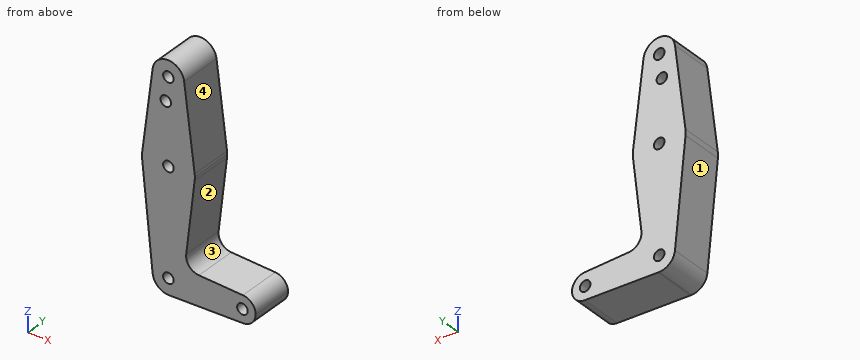
from build123d import *

# Parameters (mm, degrees)
F0_R     = 3.175
F1_DEPTH = 25.4


with BuildPart() as f1:
    # F0 (on Front) → F1 (new body)
    with BuildSketch(Plane.XZ):
        with BuildLine():
            ThreePointArc((15.769913, -1.823585), (15.848707, -0.913305), (15.875, 0))
            ThreePointArc((15.875, 0), (15.843841, 0.994139), (15.750488, 1.984375))
            ThreePointArc((15.750488, 1.984375), (0, 15.875), (-15.750488, 1.984375))
            ThreePointArc((-15.750488, 1.984375), (-15.873744, 0.199705), (-15.795426, -1.5875))
            ThreePointArc((-15.795426, -1.5875), (-0.11873, -15.874556), (15.769913, -1.823585))
        make_face()
        Circle(F0_R, mode=Mode.SUBTRACT)
        with BuildLine():
            ThreePointArc((-15.750488, 1.984375), (0, 15.875), (15.750488, 1.984375))
            Line((15.750488, 1.984375), (9.450293, 51.990625))
            ThreePointArc((9.450293, 51.990625), (9.506305, 51.396483), (9.525, 50.8))
            ThreePointArc((9.525, 50.8), (-0.596483, 41.293695), (-9.450293, 51.990625))
            Line((-9.450293, 51.990625), (-15.750488, 1.984375))
        make_face()
        with Locations((-1.5875, 36.5252)):
            Circle(F0_R, mode=Mode.SUBTRACT)
        with BuildLine():
            Line((10.688919, -45.762768), (15.769913, -1.823585))
            ThreePointArc((15.769913, -1.823585), (-0.11873, -15.874556), (-15.795426, -1.5875))
            Line((-15.795426, -1.5875), (-9.477255, -64.4525))
            ThreePointArc((-9.477255, -64.4525), (-0.476848, -53.986944), (9.525, -63.5))
            ThreePointArc((9.525, -63.5), (6.970557, -69.991299), (0.677344, -73.000886))
            Line((0.677344, -73.000886), (44.732405, -71.432475))
            ThreePointArc((44.732405, -71.432475), (36.5125, -63.5), (44.732405, -55.567525))
            Line((44.732405, -55.567525), (18.303005, -54.626608))
            ThreePointArc((18.303005, -54.626608), (12.555174, -51.861835), (10.688919, -45.762768))
        make_face()
        with BuildLine():
            ThreePointArc((9.525, 50.8), (9.506305, 51.396483), (9.450293, 51.990625))
            ThreePointArc((9.450293, 51.990625), (0, 60.325), (-9.450293, 51.990625))
            ThreePointArc((-9.450293, 51.990625), (-0.596483, 41.293695), (9.525, 50.8))
        make_face()
        with Locations((0, 50.8)):
            Circle(F0_R, mode=Mode.SUBTRACT)
        with BuildLine():
            ThreePointArc((9.525, -63.5), (-0.476848, -53.986944), (-9.477255, -64.4525))
            ThreePointArc((-9.477255, -64.4525), (-6.389564, -70.563929), (0, -73.025))
            Line((0, -73.025), (0.677344, -73.000886))
            ThreePointArc((0.677344, -73.000886), (6.970557, -69.991299), (9.525, -63.5))
        make_face()
        with Locations((0, -63.5)):
            Circle(F0_R, mode=Mode.SUBTRACT)
        with BuildLine():
            Line((0.677344, -73.000886), (0, -73.025))
            ThreePointArc((0, -73.025), (0.338886, -73.01897), (0.677344, -73.000886))
        make_face()
        with BuildLine():
            ThreePointArc((52.3875, -63.5), (50.161633, -57.98809), (44.732405, -55.567525))
            ThreePointArc((44.732405, -55.567525), (36.5125, -63.5), (44.732405, -71.432475))
            ThreePointArc((44.732405, -71.432475), (50.161633, -69.01191), (52.3875, -63.5))
        make_face()
        with Locations((44.45, -63.5)):
            Circle(F0_R, mode=Mode.SUBTRACT)
    extrude(amount=F1_DEPTH)


solid = f1.part
Model file for the job. Use its own axes, mm. Face numbers are marked on the shaded views. Give positions to 0.01 mm unless a question says otherwise; leave off trailing zeros. Loops run counter-clockwise (first coordinate to the right, second up) from the corner with the lowest first, then second, coordinate; pieces in that order, holes last. Notation, with made-up numbers: (38, 61) -> (59, 61) arc R30 ccw to (59, 85) -> close; hole circle Ø2 at (-0.5, 53.5). An arc over 180 degrees is marked (long way). Use a Markdown table: item, result. Add a question column.
(1) Slice it at A-A on y = -7. Give the number of separate pieces and of enclosed holes in the cut face, and give its area (3 significant figures).
(2) Mould opens along Z. For the marked faces 1, 2, 3 and 4 say: +Z half, -Z half, draft (parallel to the pull), parting line (faces both ways), or undercut.
(3) Drop flat-ended pins along their axis: pin 1 Ø5 at (y, z) = (-21, 38) entering from +X; pin 2 Ø1 at (y, z) = (-18, -48.5) entering from -X; pin 3 Ø2 at (x, y) = (36.5, -6.5) entering from -Z. Give the stop position or say it passes through.
(4) Slice it at B-B on z = 44.5. List the corners of the cut face in (x, y).
(5) Slice it at C-C on x = 38.5. List the corners of the cut face in (y, z), and give its area (3 significant figures).
(6) Wall check: line 1 along Z through (x, y) = (44.45, -16.5) (3 decimals); line 2 along X through (y, z) = (-17.75, -62); line 3 along X through (y, z) = (-7, 34). Give the ranges that are in metal, low to high.
Filled sheet:
| question | item | result |
|---|---|---|
| 1 | separate pieces | 1 |
| 1 | enclosed holes | 5 |
| 1 | area | 3,750 mm2 |
| 2 | face 1 | -Z half |
| 2 | face 2 | undercut |
| 2 | face 3 | undercut |
| 2 | face 4 | +Z half |
| 3 | pin 1 | x = 11.53 |
| 3 | pin 2 | x = -11.13 |
| 3 | pin 3 | z = -71.76 |
| 4 | outline | (-10.39, -25.4) -> (10.39, -25.4) -> (10.39, 0) -> (-10.39, 0) -> close |
| 5 | outline | (-25.4, -71.65) -> (0, -71.65) -> (0, -55.35) -> (-25.4, -55.35) -> close |
| 5 | area | 414 mm2 |
| 6 | line 1 | -71.443 to -66.675, -60.325 to -55.557 |
| 6 | line 2 | -9.72 to -2.8, 2.8 to 41.65, 47.25 to 52.24 |
| 6 | line 3 | -11.72 to -3.51, 0.34 to 11.72 |
